Design review of the part built by this model. Coordinates are the model's own, in mm. Face numbers are marked on the shaded views. A direction names the side the tool comes from. Round coordinates to 2 decimals unless told otherwise and drop trailing zeros. Loops run counter-clockwise (first coordinate to the right, second up) from the corner with the lowest first, then second, coordinate; pieces in that order, holes last. Notation, with made-up numbers: (66.5, -31) - (93.5, -31) arc R20 ccw to (93.5, -13) - close; hole circle Ø10 at (-29, 73.25). An arc over 180 degrees is marked (long way). Return JSON: item names as keys, results as strings. Group by question number.
(1) Wall thickness on L1, parallel to Z at x = 5, y = 0; L2, parallel to Z at x = 7.5, y = 1; L3, parallel to Y at x = 45, z = -2: over which ranges is each line inside the solid? List them lowest first. Write a range as [from, to].
(2) For the marked faces 1 and 2, list the 3-axis set-ups (+Z, -Z, +X, -X, +Y, -Y) from which the entire face can be reached by the end or side of a thin tool; tool diameter is ignored.
(3) We need section C-C, the plane z = -34.5. Write out the cut boundary in (x, y), and give its area (3 significant figures).
(4) We need section B-B, the plane y = 3.25. Write out the cut boundary in (x, z).
(5) We need section A-A, the plane z = -5. Write out the cut boundary in (x, y), and give its area (3 significant figures).
(6) Clearance check with flat-ended pins moving along their axes: pin 1 (2.5 mm diameter, centred on x = 12, y = 0, fed in from +Z); pin 2 (4 mm diameter, centred on x = 45, y = 0, fed in from +Z); pin 3 (5 mm diameter, centred on x = 45.5, y = 2.5, fed in from -Z). State where each tip first meets the part, or that it passes through.
from build123d import *

# Parameters (mm, degrees)
BOSS_EXTRUDE1_DEPTH                  = 4.7625
TAP_DRILL_FOR_M5X0_8_TAP1_AT_2_COUNT = 2
TAP_DRILL_FOR_M5X0_8_TAP1_AT_2_PITCH = 33


with BuildPart() as part:
    # Sketch1 → Boss-Extrude1 (new, symmetric)
    with BuildSketch(Plane(origin=(0, 0, 0), x_dir=(1, 0, 0), z_dir=(0, 1, 0))):
        Polygon((0, 0), (50, 0), (50, 10), (35.254833996, 10), (10, 35.254833996), (10, 50), (0, 50), align=None)
    extrude(amount=BOSS_EXTRUDE1_DEPTH, both=True)

    # Sketch6 → Tap Drill for M5x0.8 Tap1 (revolve, cut)
    with BuildSketch(Plane(origin=(12, 0, 0), x_dir=(0, -1, 0), z_dir=(1, 0, 0))):
        Polygon((0, 0), (0, 9.2618073), (2.1, 8), (2.1, 0.025), (2.125, 0), align=None)
    tap_drill_for_m5x0_8_tap1 = revolve(axis=Axis((12, 0, 6.35), (0, 0, -1)), mode=Mode.SUBTRACT)

    # Tap Drill for M5x0.8 Tap1 at 2: Tap Drill for M5x0.8 Tap1 ×2
    with Locations(*[(i * TAP_DRILL_FOR_M5X0_8_TAP1_AT_2_PITCH, 0, 0) for i in range(1, TAP_DRILL_FOR_M5X0_8_TAP1_AT_2_COUNT)]):
        add(tap_drill_for_m5x0_8_tap1, mode=Mode.SUBTRACT)

    # Mirror1: Tap Drill for M5x0.8 Tap1 across plane
    add(tap_drill_for_m5x0_8_tap1.mirror(Plane(origin=(0, 0, 0), x_dir=(-0.7071067811865478, 0, 0.7071067811865472), z_dir=(0.7071067811865475, 0, 0.7071067811865477))), mode=Mode.SUBTRACT)

    # Mirror1 copy 1 sketch → Mirror1 copy 1 (revolve, cut)
    with BuildSketch(Plane(origin=(0, 0, -45), x_dir=(0, -1, 0), z_dir=(0, 0, -1))):
        Polygon((0, 0), (0, -9.2618073), (2.1, -8), (2.1, -0.025), (2.125, 0), align=None)
    revolve(axis=Axis((-6.35, 0, -45), (-1, 0, 0)), mode=Mode.SUBTRACT)

    # Sketch10 → Tap Drill for M5x0.8 Tap2 (revolve, cut)
    with BuildSketch(Plane(origin=(15.556349186, 4.7625, -15.556349186), x_dir=(0, 0, 1), z_dir=(1, 0, 0))):
        Polygon((0, 0), (0, 9.525), (2.125, 9.525), (2.1, 9.5), (2.1, 0.025), (2.125, 0), align=None)
    revolve(axis=Axis((15.556349186, 11.1125, -15.556349186), (0, -1, 0)), mode=Mode.SUBTRACT)


solid = part.part
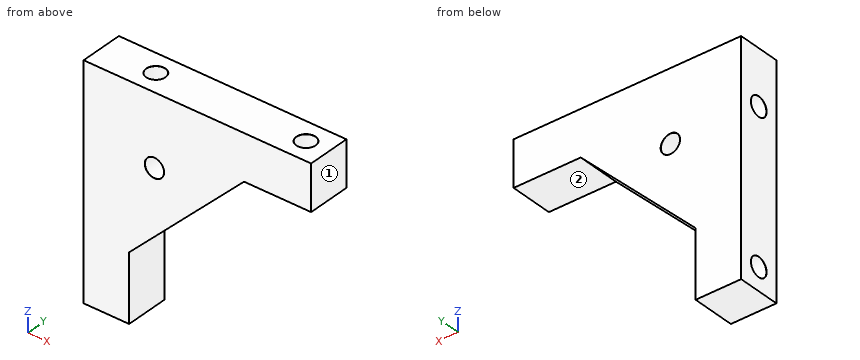
Solutions:
{
 "1": {"L1": "[-50, -47.1], [-42.9, -14.1], [-9.9, 0]", "L2": "[-50, -46.85], [-43.15, -13.85], [-10.15, 0]", "L3": "[-4.76, -2.1], [2.1, 4.76]"},
 "2": {"face 1": "+Z, -Z, +X, +Y, -Y", "face 2": "-Z, +X, +Y, -Y"},
 "3": {"outline": "(0, -4.76) - (10.75, -4.76) - (10.75, 4.76) - (0, 4.76) - close", "area": "102 mm^2"},
 "4": {"outline": "(0, -50) - (10, -50) - (10, -35.25) - (35.25, -10) - (50, -10) - (50, 0) - (0, 0) - close; hole circle Ø4.2 at (15.56, -15.56)"},
 "5": {"outline": "(0, -4.76) - (50, -4.76) - (50, 4.76) - (0, 4.76) - close; hole circle Ø4.2 at (12, 0); hole circle Ø4.2 at (45, 0)", "area": "449 mm^2"},
 "6": {"pin 1": "z = -8.51", "pin 2": "z = -8.06", "pin 3": "z = -10"}
}
